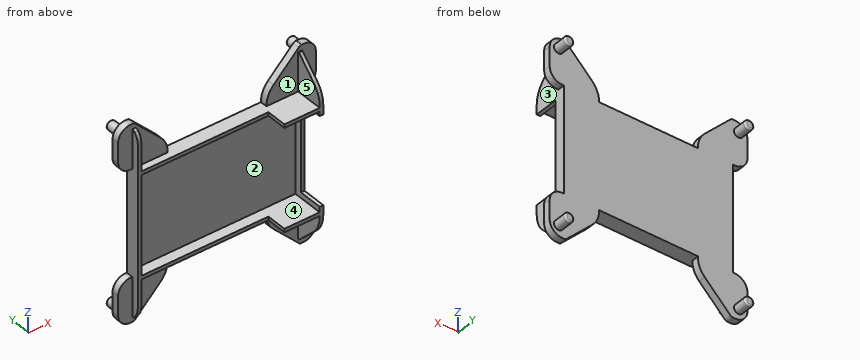
```python
from build123d import *

# Parameters (mm, degrees)
SKETCH_W        = 96
SKETCH_H        = 60
PAD_DEPTH       = 30
SKETCH001_W     = 92
SKETCH001_H     = 56
POCKET_DEPTH    = 28
SKETCH002_W     = 74
SKETCH002_H     = 22
POCKET001_DEPTH = 60
SKETCH003_W     = 22
SKETCH003_H     = 4
POCKET002_DEPTH = 60
SKETCH005_W     = 22
SKETCH005_H     = 6.4
POCKET003_DEPTH = 60
SKETCH004_W     = 50.3
SKETCH004_H     = 13.6
POCKET004_DEPTH = 5
SKETCH006_W     = 20
SKETCH006_H     = 4
PAD001_DEPTH    = 25
SKETCH007_W     = 20
SKETCH007_H     = 4
PAD002_DEPTH    = 25
SKETCH008_W     = 25
SKETCH008_H     = 4
PAD003_DEPTH    = 8
SKETCH009_W     = 25
SKETCH009_H     = 4
PAD004_DEPTH    = 8
SKETCH010_R     = 2.6
PAD005_DEPTH    = 8
FILLET_R        = 1
FILLET001_R     = 1
FILLET002_R     = 1
FILLET003_R     = 1
CHAMFER_SIZE    = 19
FILLET004_R     = 7
FILLET005_R     = 2
FILLET006_R     = 13
FILLET007_R     = 7
CHAMFER001_SIZE = 19
FILLET008_R     = 14
FILLET009_R     = 2
FILLET010_R     = 7
FILLET011_R     = 7
CHAMFER002_SIZE = 19
FILLET012_R     = 13
FILLET013_R     = 2
FILLET014_R     = 7
FILLET015_R     = 7
FILLET016_R     = 7
FILLET017_R     = 7
CHAMFER003_SIZE = 19
FILLET018_R     = 2
FILLET019_R     = 13
SKETCH011_W     = 2
SKETCH011_H     = 15.6
SKETCH011_H_2   = 4
PAD006_DEPTH    = 22
CHAMFER004_SIZE = 15
FILLET020_R     = 15
CHAMFER005_SIZE = 3
FILLET021_R     = 2
FILLET022_R     = 8
SKETCH012_W     = 2
SKETCH012_H     = 15.6
SKETCH012_H_2   = 4
PAD007_DEPTH    = 22
CHAMFER006_SIZE = 15
FILLET023_R     = 16
FILLET024_R     = 1
CHAMFER007_SIZE = 3
FILLET025_R     = 10


with BuildPart() as part:
    # Sketch → Pad (new body)
    with BuildSketch(Plane.XZ):
        with Locations((-0.226995, -30.10394)):
            Rectangle(SKETCH_W, SKETCH_H)
    extrude(amount=PAD_DEPTH)

    # Sketch001 (on Face6 of Pad) → Pocket (cut)
    with BuildSketch(Plane.XZ.offset(30)):
        with Locations((-0.226995, -30.10394)):
            Rectangle(SKETCH001_W, SKETCH001_H)
    extrude(amount=-POCKET_DEPTH, mode=Mode.SUBTRACT)

    # Sketch002 (on Face6 of Pocket) → Pocket001 (cut)
    with BuildSketch(Plane(origin=(0, 0, -60.10394), x_dir=(1, 0, 0), z_dir=(0, 0, -1))):
        with Locations((-11.226995, 19)):
            Rectangle(SKETCH002_W, SKETCH002_H)
    extrude(amount=-POCKET001_DEPTH, mode=Mode.SUBTRACT)

    # Sketch003 (on Face8 of Pocket001) → Pocket002 (cut)
    with BuildSketch(Plane(origin=(0, 0, -60.10394), x_dir=(1, 0, 0), z_dir=(0, 0, -1))):
        with Locations((36.773005, 28)):
            Rectangle(SKETCH003_W, SKETCH003_H)
    extrude(amount=-POCKET002_DEPTH, mode=Mode.SUBTRACT)

    # Sketch005 (on Face8 of Pocket002) → Pocket003 (cut)
    with BuildSketch(Plane(origin=(0, 0, -60.10394), x_dir=(1, 0, 0), z_dir=(0, 0, -1))):
        with Locations((36.773005, 22.8)):
            Rectangle(SKETCH005_W, SKETCH005_H)
    extrude(amount=-POCKET003_DEPTH, mode=Mode.SUBTRACT)

    # Sketch004 (on Face3 of Pocket002) → Pocket004 (cut)
    with BuildSketch(Plane(origin=(47.773005, 0, 0), x_dir=(0, 0, 1), z_dir=(1, 0, 0))):
        with Locations((-29.85394, 12.8)):
            Rectangle(SKETCH004_W, SKETCH004_H)
    extrude(amount=-POCKET004_DEPTH, mode=Mode.SUBTRACT)

    # Sketch006 (on Face1 of Pocket004) → Pad001 (join)
    with BuildSketch(Plane(origin=(0, 0, -0.10394), x_dir=(-1, 0, 0), z_dir=(0, 0, 1))):
        with Locations((-37.773005, 2)):
            Rectangle(SKETCH006_W, SKETCH006_H)
        with Locations((38.226995, 2)):
            Rectangle(SKETCH006_W, SKETCH006_H)
    extrude(amount=PAD001_DEPTH)

    # Sketch007 (on Face14 of Pad001) → Pad002 (join)
    with BuildSketch(Plane(origin=(0, 0, -60.10394), x_dir=(1, 0, 0), z_dir=(0, 0, -1))):
        with Locations((-38.226995, 2)):
            Rectangle(SKETCH007_W, SKETCH007_H)
        with Locations((37.773005, 2)):
            Rectangle(SKETCH007_W, SKETCH007_H)
    extrude(amount=PAD002_DEPTH)

    # Sketch008 (on Face19 of Pad002) → Pad003 (join)
    with BuildSketch(Plane(origin=(47.773005, 0, 0), x_dir=(0, 0, 1), z_dir=(1, 0, 0))):
        with Locations((-72.60394, 2)):
            Rectangle(SKETCH008_W, SKETCH008_H)
        with Locations((12.5, 2)):
            Rectangle(SKETCH008_W, SKETCH008_H)
    extrude(amount=PAD003_DEPTH)

    # Sketch009 (on Face31 of Pad003) → Pad004 (join)
    with BuildSketch(Plane(origin=(-48.226995, 0, 0), x_dir=(0, 0, -1), z_dir=(-1, 0, 0))):
        with Locations((-12.39606, 2)):
            Rectangle(SKETCH009_W, SKETCH009_H)
        with Locations((72.60394, 2)):
            Rectangle(SKETCH009_W, SKETCH009_H)
    extrude(amount=PAD004_DEPTH)

    # Sketch010 (on Face2 of Pad004) → Pad005 (join)
    with BuildSketch(Plane(origin=(0, 0, 0), x_dir=(1, 0, 0), z_dir=(0, 1, 0))):
        with Locations((50.773005, 79.10394)):
            Circle(SKETCH010_R)
        with Locations((50.773005, -19)):
            Circle(SKETCH010_R)
        with Locations((-51.226995, -18.89606)):
            Circle(SKETCH010_R)
        with Locations((-51.226995, 79.10394)):
            Circle(SKETCH010_R)
    extrude(amount=PAD005_DEPTH)

    # Fillet
    fillet_edges = [part.edges().sort_by_distance(p)[0] for p in [
        (48.173005, 8, 19),
    ]]
    fillet(fillet_edges, radius=FILLET_R)

    # Fillet001
    fillet001_edges = [part.edges().sort_by_distance(p)[0] for p in [
        (48.173005, 8, -79.10394),
    ]]
    fillet(fillet001_edges, radius=FILLET001_R)

    # Fillet002
    fillet002_edges = [part.edges().sort_by_distance(p)[0] for p in [
        (-53.826995, 8, -79.10394),
    ]]
    fillet(fillet002_edges, radius=FILLET002_R)

    # Fillet003
    fillet003_edges = [part.edges().sort_by_distance(p)[0] for p in [
        (-53.826995, 8, 18.89606),
    ]]
    fillet(fillet003_edges, radius=FILLET003_R)

    # Chamfer
    chamfer_edges = [part.edges().sort_by_distance(p)[0] for p in [
        (27.773005, -2, -85.10394),
    ]]
    chamfer(chamfer_edges, length=CHAMFER_SIZE)

    # Fillet004
    fillet004_edges = [part.edges().sort_by_distance(p)[0] for p in [
        (55.773005, -2, -85.10394),
    ]]
    fillet(fillet004_edges, radius=FILLET004_R)

    # Fillet005
    fillet005_edges = [part.edges().sort_by_distance(p)[0] for p in [
        (46.773005, -2, -85.10394),
    ]]
    fillet(fillet005_edges, radius=FILLET005_R)

    # Fillet006
    fillet006_edges = [part.edges().sort_by_distance(p)[0] for p in [
        (27.773005, -2, -66.10394),
    ]]
    fillet(fillet006_edges, radius=FILLET006_R)

    # Fillet007
    fillet007_edges = [part.edges().sort_by_distance(p)[0] for p in [
        (55.773005, -2, -60.10394),
    ]]
    fillet(fillet007_edges, radius=FILLET007_R)

    # Chamfer001
    chamfer001_edges = [part.edges().sort_by_distance(p)[0] for p in [
        (27.773005, -2, 24.89606),
    ]]
    chamfer(chamfer001_edges, length=CHAMFER001_SIZE)

    # Fillet008
    fillet008_edges = [part.edges().sort_by_distance(p)[0] for p in [
        (27.773005, -2, 5.89606),
    ]]
    fillet(fillet008_edges, radius=FILLET008_R)

    # Fillet009
    fillet009_edges = [part.edges().sort_by_distance(p)[0] for p in [
        (46.773005, -2, 24.89606),
    ]]
    fillet(fillet009_edges, radius=FILLET009_R)

    # Fillet010
    fillet010_edges = [part.edges().sort_by_distance(p)[0] for p in [
        (55.773005, -2, 25),
    ]]
    fillet(fillet010_edges, radius=FILLET010_R)

    # Fillet011
    fillet011_edges = [part.edges().sort_by_distance(p)[0] for p in [
        (55.773005, -2, 0),
    ]]
    fillet(fillet011_edges, radius=FILLET011_R)

    # Chamfer002
    chamfer002_edges = [part.edges().sort_by_distance(p)[0] for p in [
        (-28.226995, -2, 24.89606),
    ]]
    chamfer(chamfer002_edges, length=CHAMFER002_SIZE)

    # Fillet012
    fillet012_edges = [part.edges().sort_by_distance(p)[0] for p in [
        (-28.226995, -2, 5.89606),
    ]]
    fillet(fillet012_edges, radius=FILLET012_R)

    # Fillet013
    fillet013_edges = [part.edges().sort_by_distance(p)[0] for p in [
        (-47.226995, -2, 24.89606),
    ]]
    fillet(fillet013_edges, radius=FILLET013_R)

    # Fillet014
    fillet014_edges = [part.edges().sort_by_distance(p)[0] for p in [
        (-56.226995, -2, 24.89606),
    ]]
    fillet(fillet014_edges, radius=FILLET014_R)

    # Fillet015
    fillet015_edges = [part.edges().sort_by_distance(p)[0] for p in [
        (-56.226995, -2, -0.10394),
    ]]
    fillet(fillet015_edges, radius=FILLET015_R)

    # Fillet016
    fillet016_edges = [part.edges().sort_by_distance(p)[0] for p in [
        (-56.226995, -2, -60.10394),
    ]]
    fillet(fillet016_edges, radius=FILLET016_R)

    # Fillet017
    fillet017_edges = [part.edges().sort_by_distance(p)[0] for p in [
        (-56.226995, -2, -85.10394),
    ]]
    fillet(fillet017_edges, radius=FILLET017_R)

    # Chamfer003
    chamfer003_edges = [part.edges().sort_by_distance(p)[0] for p in [
        (-28.226995, -2, -85.10394),
    ]]
    chamfer(chamfer003_edges, length=CHAMFER003_SIZE)

    # Fillet018
    fillet018_edges = [part.edges().sort_by_distance(p)[0] for p in [
        (-47.226995, -2, -85.10394),
    ]]
    fillet(fillet018_edges, radius=FILLET018_R)

    # Fillet019
    fillet019_edges = [part.edges().sort_by_distance(p)[0] for p in [
        (-28.226995, -2, -66.10394),
    ]]
    fillet(fillet019_edges, radius=FILLET019_R)

    # Sketch011 (on Face13 of Fillet019) → Pad006 (join)
    with BuildSketch(Plane(origin=(0, 0, -0.10394), x_dir=(-1, 0, 0), z_dir=(0, 0, 1))):
        with Locations((-46.773005, 11.8)):
            Rectangle(SKETCH011_W, SKETCH011_H)
        with Locations((47.226995, 6)):
            Rectangle(SKETCH011_W, SKETCH011_H_2)
    extrude(amount=PAD006_DEPTH)

    # Chamfer004
    chamfer004_edges = [part.edges().sort_by_distance(p)[0] for p in [
        (46.773005, -19.6, 21.89606),
    ]]
    chamfer(chamfer004_edges, length=CHAMFER004_SIZE)

    # Fillet020
    fillet020_edges = [part.edges().sort_by_distance(p)[0] for p in [
        (46.773005, -19.6, 6.89606),
    ]]
    fillet(fillet020_edges, radius=FILLET020_R)

    # Chamfer005
    chamfer005_edges = [part.edges().sort_by_distance(p)[0] for p in [
        (-47.226995, -8, 21.89606),
    ]]
    chamfer(chamfer005_edges, length=CHAMFER005_SIZE)

    # Fillet021
    fillet021_edges = [part.edges().sort_by_distance(p)[0] for p in [
        (-47.226995, -5, 21.89606),
    ]]
    fillet(fillet021_edges, radius=FILLET021_R)

    # Fillet022
    fillet022_edges = [part.edges().sort_by_distance(p)[0] for p in [
        (-47.226995, -8, 18.89606),
    ]]
    fillet(fillet022_edges, radius=FILLET022_R)

    # Sketch012 (on Face24 of Fillet022) → Pad007 (join)
    with BuildSketch(Plane(origin=(0, 0, -60.10394), x_dir=(1, 0, 0), z_dir=(0, 0, -1))):
        with Locations((46.773005, 11.8)):
            Rectangle(SKETCH012_W, SKETCH012_H)
        with Locations((-47.226995, 6)):
            Rectangle(SKETCH012_W, SKETCH012_H_2)
    extrude(amount=PAD007_DEPTH)

    # Chamfer006
    chamfer006_edges = [part.edges().sort_by_distance(p)[0] for p in [
        (46.773005, -19.6, -82.10394),
    ]]
    chamfer(chamfer006_edges, length=CHAMFER006_SIZE)

    # Fillet023
    fillet023_edges = [part.edges().sort_by_distance(p)[0] for p in [
        (46.773005, -19.6, -67.10394),
    ]]
    fillet(fillet023_edges, radius=FILLET023_R)

    # Fillet024
    fillet024_edges = [part.edges().sort_by_distance(p)[0] for p in [
        (46.773005, -4.6, -82.10394),
    ]]
    fillet(fillet024_edges, radius=FILLET024_R)

    # Chamfer007
    chamfer007_edges = [part.edges().sort_by_distance(p)[0] for p in [
        (-47.226995, -8, -82.10394),
    ]]
    chamfer(chamfer007_edges, length=CHAMFER007_SIZE)

    # Fillet025
    fillet025_edges = [part.edges().sort_by_distance(p)[0] for p in [
        (-47.226995, -8, -79.10394),
    ]]
    fillet(fillet025_edges, radius=FILLET025_R)


solid = part.part
```
The listing builds one solid part. Answer for the finished solid, in the listing's coordinates (mm). Face numbers are marked on the shaded views. A direction names the side the tool comes from. Give positions to 0.01 mm unless a question says otherwise; leave off trailing zeros. Loops run counter-clockwise (first coordinate to the right, second up) from the corner with the lowest first, then second, coordinate; pieces in that order, holes last. Notation, with made-up numbers: (35, 56) - (82, 56) arc R14 cw to (82, 70) - close; hole circle Ø2 at (-16.75, 18). An arc over 180 degrees is marked (long way). Answer as CSV lines item,"result". Start each with the question number.
Item 1: A cutting plane is placed at B-B on x = -23. Determine the outline of the cut face in (y, z).
Item 2: The mould has two halves that part along Z. Classify the marked faces 1, 2 and 3: +Z half, -Z half, draft (parallel to the pull), parting line (faces both ways), or undercut.
Item 3: Each of these flat-tipped pins is pushed along its axis until it touches: pin 1 (3 mm diameter, centred on x = -28, z = 0.5, fed in from +Y); pin 2 (22 mm diameter, centred on x = -13, z = -45.5, fed in from -Y); pin 3 (7.5 mm diameter, centred on x = 35.5, z = -78.5, fed in from -Y). Where does it stop, or does it pass through?
Item 4: For the marked faces 4 and 5, determine the directions among +Z, -Z, +X, -X, +Y, -Y from which every point of the face is accessible in a straight line to the end or side of a thin tool.
Item 5: A cutting plane is placed at A-A on z = -33. Determine the outline of the cut face in (x, y).
Item 6: Find the intervals of material crossed by line 1 (Z direction, x = 42.5, y = -11); line 2 (X direction, y = -2.5, z = -32); line 3 (X direction, y = -16, z = -70.5), in increasing order. Write a range as from..to.
Found:
1,outline,"(-8, -60.1) - (0, -60.1) - (0, -0.1) - (-8, -0.1) - (-8, -2.1) - (-2, -2.1) - (-2, -58.1) - (-8, -58.1) - close"
2,face 1,"draft"
2,face 2,"undercut"
2,face 3,"undercut"
3,pin 1,"stops at y = 0"
3,pin 2,"stops at y = -2"
3,pin 3,"stops at y = -4"
4,face 4,"-Y"
4,face 5,"+Z, -Y"
5,outline,"(-48.23, -8) - (-46.23, -8) - (-46.23, -2) - (45.77, -2) - (45.77, -6) - (47.77, -6) - (47.77, 0) - (-48.23, 0) - close"
6,line 1,"z = -60.1..-58.1, -2.1..-0.1"
6,line 2,"x = -48.23..-46.23, 45.77..47.77"
6,line 3,"x = 45.77..47.77"
